```python
from build123d import *

# Parameters (mm, degrees)
SKETCH1_W           = 38
SKETCH1_H           = 10
SKETCH1_H_2         = 12
SKETCH1_W_2         = 12
SKETCH1_H_3         = 28
BOSS_EXTRUDE1_DEPTH = 18
SKETCH1_3_W         = 38
SKETCH1_3_H         = 12
SKETCH1_3_W_2       = 12
SKETCH1_3_H_2       = 28
SKETCH1_3_H_3       = 10
BOSS_EXTRUDE2_DEPTH = 38


with BuildPart() as part:
    # Sketch1 → Boss-Extrude1 (new body)
    with BuildSketch(Plane(origin=(0, 0, 0), x_dir=(1, 0, 0), z_dir=(0, 1, 0))):
        with Locations((25, 20)):
            Rectangle(SKETCH1_W, SKETCH1_H)
        with Locations((25, 9)):
            Rectangle(SKETCH1_W, SKETCH1_H_2)
        with Locations((0, 9)):
            Rectangle(SKETCH1_W_2, SKETCH1_H_2)
        with Locations((25, -11)):
            Rectangle(SKETCH1_W, SKETCH1_H_3)
        with Locations((0, -11)):
            Rectangle(SKETCH1_W_2, SKETCH1_H_3)
        with Locations((-25, -11)):
            Rectangle(SKETCH1_W, SKETCH1_H_3)
        with Locations((-25, 9)):
            Rectangle(SKETCH1_W, SKETCH1_H_2)
        with Locations((-25, 20)):
            Rectangle(SKETCH1_W, SKETCH1_H)
        with Locations((0, 20)):
            Rectangle(SKETCH1_W_2, SKETCH1_H)
    extrude(amount=-BOSS_EXTRUDE1_DEPTH)

    # Sketch1<3> → Boss-Extrude2 (add)
    with BuildSketch(Plane(origin=(0, 0, 0), x_dir=(1, 0, 0), z_dir=(0, 1, 0))):
        with Locations((-25, 9)):
            Rectangle(SKETCH1_3_W, SKETCH1_3_H)
        with Locations((0, 9)):
            Rectangle(SKETCH1_3_W_2, SKETCH1_3_H)
        with Locations((25, 9)):
            Rectangle(SKETCH1_3_W, SKETCH1_3_H)
        with Locations((0, -11)):
            Rectangle(SKETCH1_3_W_2, SKETCH1_3_H_2)
        with Locations((0, 20)):
            Rectangle(SKETCH1_3_W_2, SKETCH1_3_H_3)
    extrude(amount=BOSS_EXTRUDE2_DEPTH)

    # SurfaceCut5
    split(bisect_by=Plane(origin=(17, 17, 17), x_dir=(0.8164965809277277, -0.4082482904638635, -0.4082482904638593), z_dir=(0.5773502691896235, 0.57735026918963, 0.577350269189624)), keep=Keep.BOTTOM)


solid = part.part
```
Geometry check sheet. Reference: the model listing, model coordinates, mm. A direction names the side the tool comes from. Round coordinates to 2 decimals unless told otherwise and drop trailing zeros. Loops run counter-clockwise (first coordinate to the right, second up) from the corner with the lowest first, then second, coordinate; pieces in that order, holes last. Notation, with made-up numbers: (52.5, 25.25) -> (94.5, 25.25) arc R31 ccw to (94.5, 54.25) -> close; hole circle Ø5 at (-2, -7.75). An arc over 180 degrees is marked (long way). Use a Markdown table: item, result.
(1) Go/stop test with flat-tipped pins: P1, Ø19, axis at x = -33, y = 22, coming from the +Z side; P2, Ø5, axis at y = 27.5, z = -20, coming from the -X side; P3, Ø5, axis at y = 19, z = -18, coming from the +X side. Record where each tip stops, or that it passes through.
Calculated:
| item | result |
|---|---|
| P1 | z = -3 |
| P2 | x = -6 |
| P3 | x = 6 |
(2) Sectioned sample at D-D (z = -2). Enter the section's corners in (x, y).
Calculated:
| item | result |
|---|---|
| outline | (-44, -18) -> (44, -18) -> (44, 0) -> (6, 0) -> (6, 38) -> (-6, 38) -> (-6, 0) -> (-44, 0) -> close |
(3) Scan lines: probe 1 along Y at (x, z) = (10.5, -19.5); probe 2 along X at (y, z) = (9, 2); probe 3 along Z at (x, y) = (-39, 22). Record each from-to range of solid material in increasing order.
Calculated:
| item | result |
|---|---|
| probe 1 | -18 to 0 |
| probe 2 | -6 to 6 |
| probe 3 | -15 to -3 |
(4) Set-up check for faces 1 (the flat face through (-25, 19, -3)), 2 (the flat face through (21, 0, 11)), 3 (the flat face through (6, 19, -20)): record each of +Z, -Z, +X, -X, +Y, -Y from which the full face is reachable in a straight line by a thin tool's end or side.
Calculated:
| item | result |
|---|---|
| face 1 | +Z, -X, +Y |
| face 2 | +Z, +X, +Y |
| face 3 | -Z, +X, +Y |
(5) Sectioned sample at B-B (y = 21). Enter the section's corners in (x, z).
Calculated:
| item | result |
|---|---|
| outline | (-44, -15) -> (-6, -15) -> (-6, -25) -> (6, -25) -> (6, -15) -> (44, -15) -> (44, -14) -> (33, -3) -> (6, -3) -> (6, 24) -> (5, 25) -> (-6, 25) -> (-6, -3) -> (-44, -3) -> close |
(6) Sectioned sample at A-A (z = 18). Enter the section's corners in (x, y), then the cut area to 3 significant figures.
Calculated:
| item | result |
|---|---|
| outline | (-44, -18) -> (44, -18) -> (44, -11) -> (33, 0) -> (6, 0) -> (6, 27) -> (-5, 38) -> (-6, 38) -> (-6, 0) -> (-44, 0) -> close |
| area | 1,920 mm² |
(7) Sectioned sample at C-C (x = 10). Enter the section's corners in (y, z).
Calculated:
| item | result |
|---|---|
| outline | (-18, -25) -> (0, -25) -> (0, -15) -> (38, -15) -> (38, -3) -> (0, -3) -> (0, 25) -> (-18, 25) -> close |
